The model under review builds one solid part; all positions refer to its coordinate system, in mm. A direction names the side the tool comes from. Give positions to 0.01 mm unless a question says otherwise; leave off trailing zeros. Order: outer loops, then holes, each group sorted by start corner. A loop starts at its lowest first (then second) coordinate and runs counter-clockwise, first axis right, second up. Notation, with made-up numbers: (-18.75, 41) - (-3.75, 41) arc R32 cw to (-3.75, 71) - close; hole circle Ø4 at (43.5, 55). An arc over 180 degrees is marked (long way). Use CSV: the item, a comma, the result in double quotes.
Autodesk Inventor part; units mm, degrees
ref_plane "YZ Plane" through (0, 0, 0) normal (1, 0, 0) x (0, 1, 0)
ref_plane "XZ Plane" through (0, 0, 0) normal (0, 1, 0) x (-1, 0, 0)
ref_plane "XY Plane" through (0, 0, 0) normal (0, 0, 1) x (1, 0, 0)
sketch "スケッチ1" plane through (0, 0, 0) normal (0, 0, 1) x (1, 0, 0)
  line L0 (102.5, -16.5) -> (-102.5, -16.5)
  line L1 (-102.5, -16.5) -> (-102.5, 16.5)
  line L2 (-102.5, 16.5) -> (102.5, 16.5)
  line L3 (102.5, 16.5) -> (102.5, -16.5)
  line L4 (102.5, -16.5) -> (-102.5, 16.5) construction
  line L5 (-102.5, -16.5) -> (102.5, 16.5) construction
  point P0 (0, 0)
  dimension "d0" = 205
  dimension "d1" = 33
extrude "プレート1" add sketch "スケッチ1" along normal blind 1.5
sketch "スケッチ2" plane through (102.5, 16.5, 0) normal (0, 0.5, 0.8660254) x (-1, 0, 0)
  line L0 (205, 0) -> (0, 0)
  line L1 (0, 0) -> (0, -20)
  line L2 (0, -20) -> (205, -20)
  line L3 (205, -20) -> (205, 0)
edge flange "フランジ1" height 20 angle 30 thickness 1.5 bend radius 1.5 thickness toward (0, 0.5, 0.8660254) relief tear relief width 1.5 relief depth 0.75 edges at (0, 16.5, 0) wall of the first edge with corners at (-102.5, 16.5, 0) (102.5, 16.5, 0) (102.5, 33.8205, -10) (-102.5, 33.8205, -10)
bend "曲げ1"
corner "コーナー1"
sketch "スケッチ3" plane through (0, 0, 1.5) normal (0, 0, 1) x (1, 0, 0)
  line L0 (102.5, 16.0981) -> (-102.5, 16.0981)
  line L1 (-102.5, -16.5) -> (-102.5, 16.0981)
  line L2 (102.5, -16.5) -> (-102.5, -16.5)
  line L3 (102.5, 16.0981) -> (102.5, -16.5)
  point P0 (0, 0)
  point P1 (-92.5, -6.5)
  point P2 (92.5, -6.5)
  point P3 (-32.5, -6.5)
  point P4 (32.5, -6.5)
  dimension "d13" = 10
  dimension "d14" = 10
  dimension "d15" = 10
  dimension "d16" = 185
  dimension "d32" = 60
  dimension "d33" = 60
hole "穴1" at (-92.5, -6.5, 1.5) at (92.5, -6.5, 1.5) at (-32.5, -6.5, 1.5) at (32.5, -6.5, 1.5) direction (0, 0, -1) diameter 4.5 end through all
fillet "フィレット1" radius 2 4 edges at (-102.5, -16.5, 0.75) (-102.5, 34.1955, -9.3505) (102.5, 34.1955, -9.3505) (102.5, -16.5, 0.75)
sketch "スケッチ4" plane through (0, 0, 1.5) normal (0, 0, 1) x (1, 0, 0)
  circle A0 centre (-32.5, -6.5) radius 2.25
  circle A1 centre (-92.5, -6.5) radius 2.25
  circle A2 centre (92.5, -6.5) radius 2.25
  circle A3 centre (32.5, -6.5) radius 2.25
  arc A4 (100.5, -16.5) -> (102.5, -14.5) centre (100.5, -14.5) ccw
  line L0 (102.5, 16.0981) -> (102.5, -14.5)
  line L1 (102.5, 16.0981) -> (-102.5, 16.0981)
  line L2 (-102.5, -14.5) -> (-102.5, 16.0981)
  arc A5 (-102.5, -14.5) -> (-100.5, -16.5) centre (-100.5, -14.5) ccw
  line L3 (100.5, -16.5) -> (-100.5, -16.5)
  line L4 (-92.5, -4) -> (-92.5, -9) construction
  line L5 (-94.75, -4) -> (-94.75, -9)
  line L6 (-90.25, -9) -> (-90.25, -4)
  arc A6 (-90.25, -4) -> (-94.75, -4) centre (-92.5, -4) ccw
  arc A7 (-94.75, -9) -> (-90.25, -9) centre (-92.5, -9) ccw
  line L7 (-32.5, -9) -> (-32.5, -4) construction
  line L8 (-30.25, -9) -> (-30.25, -4)
  line L9 (-34.75, -4) -> (-34.75, -9)
  arc A8 (-34.75, -9) -> (-30.25, -9) centre (-32.5, -9) ccw
  arc A9 (-30.25, -4) -> (-34.75, -4) centre (-32.5, -4) ccw
  line L10 (32.5, -9) -> (32.5, -4) construction
  circle A10 centre (32.5, -6.5) radius 2.25
  line L11 (30.25, -9) -> (30.25, -4)
  line L12 (34.75, -4) -> (34.75, -9)
  arc A11 (30.25, -9) -> (34.75, -9) centre (32.5, -9) ccw
  arc A12 (34.75, -4) -> (30.25, -4) centre (32.5, -4) ccw
  line L13 (92.5, -9) -> (92.5, -4) construction
  line L14 (90.25, -9) -> (90.25, -4)
  line L15 (94.75, -4) -> (94.75, -9)
  arc A13 (90.25, -9) -> (94.75, -9) centre (92.5, -9) ccw
  arc A14 (94.75, -4) -> (90.25, -4) centre (92.5, -4) ccw
  circle A15 centre (-32.5, -6.5) radius 2.25
  circle A16 centre (-92.5, -6.5) radius 2.25
  point P0 (0, 0)
  dimension "d34" = 5
extrude "押し出し1" cut sketch "スケッチ4" against normal blind 10 contours A0 | L8 A8 L9 A0 | A0 L9 A9 L8 | A1 | L6 A7 L5 A1 | A1 L5 A6 L6 | A2 | L15 A13 L14 A2 | A2 L14 A14 L15 | A3 | L12 A11 L11 A3 | A3 L11 A12 L12
equation "\"d29\" = Thickness"
equation "\"d2\" = Thickness"
equation "\"d3\" = BendReliefWidth"
equation "\"d4\" = BendReliefDepth"
equation "\"d5\" = MinimumRemnant"
equation "\"d6\" = TransitionRadius"
equation "\"d9\" = BendRadius"
equation "\"d10\" = CornerReliefSize"
equation "\"d11\" = GapSize"
equation "\"d12\" = JacobiRadiusSize"
equation "\"BendRadius\" = Thickness"
equation "\"BendReliefWidth\" = Thickness"
equation "\"BendReliefDepth\" = 0.5 * Thickness"
equation "\"CornerReliefSize\" = 4 * Thickness"
equation "\"MinimumRemnant\" = 2 * Thickness"
equation "\"TransitionRadius\" = BendRadius"
equation "\"JacobiRadiusSize\" = BendRadius"
equation "\"GapSize\" = Thickness"
properties part number "Scraper_Bar"
Item 1: Tool access review of faces 1 (the face through (-1, 0, 0)), 2 (the face through (102.5, 11, 1)): name each direction out of +Z, -Z, +X, -X, +Y, -Y from which nothing blocks a thin tool from reaching the whole face with its end or side.
Results list:
face 1,"-Z, +X, -X, -Y"
face 2,"+Z, -Z, +X, +Y, -Y"
Item 2: Take a section at B-B, the plane x = 76.5. Give the boundary of the cut face in (y, z), and give its area (3 significant figures).
Results list:
outline,"(-16.5, 0) - (16.1, 0) arc R1.5 cw to (16.85, -0.2) - (33.82, -10) - (34.57, -8.7) - (17.6, 1.1) arc R3 ccw to (16.1, 1.5) - (-16.5, 1.5) - close"
area,"80.1 mm2"
Item 3: Take a section at D-D, the plane z = -4.25. Give the boundary of the cut face in (x, y).
Results list:
outline,"(-102.5, 23.86) - (102.5, 23.86) - (102.5, 26.86) - (-102.5, 26.86) - close"
Item 4: Clearance check with flat-ended pins moving along their axes: pin 1 (16.5 mm diameter, centred on x = 42, y = -1.5, fed in from -Z); pin 2 (1 mm diameter, centred on x = -52, z = -6, fed in from +Y); pin 3 (2 mm diameter, centred on y = 24.5, z = -0.5, fed in from +X); pin 4 (3 mm diameter, centred on y = 25.5, z = -2, fed in from -X). State where each tip first meets the part, or that it passes through.
Results list:
pin 1,"stops at z = 0"
pin 2,"stops at y = 30.76"
pin 3,"passes through"
pin 4,"stops at x = -102.5"
Item 5: Take a section at A-A, the plane x = -32.5. Give the boundary of the cut face in (y, z).
Results list:
outline,"(-16.5, 0) - (-11.25, 0) - (-11.25, 1.5) - (-16.5, 1.5) - close; (-1.75, 0) - (16.1, 0) arc R1.5 cw to (16.85, -0.2) - (33.82, -10) - (34.57, -8.7) - (17.6, 1.1) arc R3 ccw to (16.1, 1.5) - (-1.75, 1.5) - close"
Item 6: Wall thickness on L1, parallel to Z at x = 36.5, y = -2; L2, parallel to Y at x = 57, z = -8.25; L3, parallel to Z at x = -34.5, y = 29.5: over which ranges is each line inside the solid? List them lowest first.
Results list:
L1,"z = 0 to 1.5"
L2,"y = 30.79 to 33.79"
L3,"z = -7.51 to -5.77"
Item 7: Take a section at C-C, the plane y = 3. Give the boundary of the cut face in (x, z), and give its area (4 significant figures).
Results list:
outline,"(-102.5, 0) - (102.5, 0) - (102.5, 1.5) - (-102.5, 1.5) - close"
area,"307.5 mm2"
